Could you check a few things on this drawing? It's one solid part, dimensions in mm from its lowest x, y, z. Round coordinates to 2 decimals unless told otherwise and drop trailing zeros. Order: outer loops, then holes, each group sorted by start corner. A loop starts at its lowest first (then second) coordinate and runs counter-clockwise, first axis right, second up. Notation, with made-up numbers: M 30.25,76 L 60.25,76 A12 ccw 60.25,82 Z; hole C 0,-29 d10. An arc over 180 degrees is marked long. Answer as a JSON object with one key per item and string values. Group by question number.
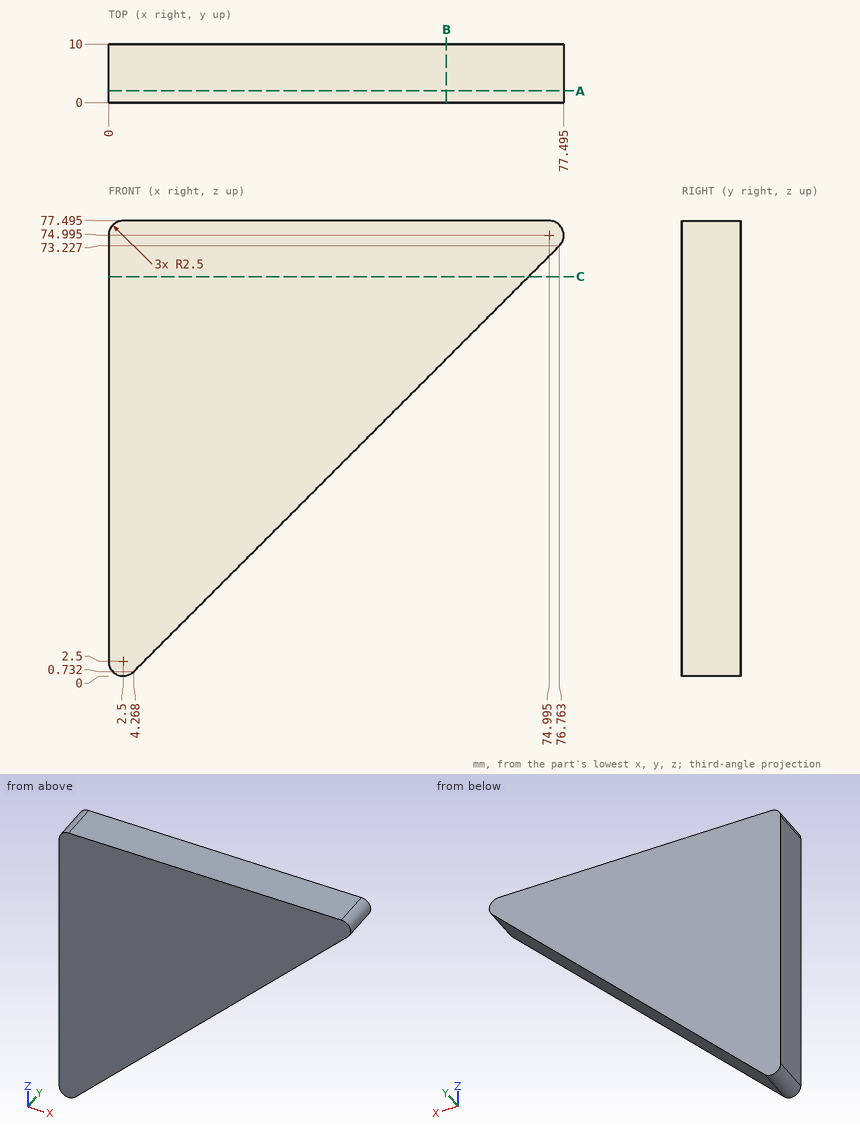
1) If we section it at C-C on z = 68: Write out the boundary of the cut face in (x, y) (1 decimal).
2) If we section it at B-B on x = 57.5: Write out the boundary of the cut face in (y, z) (1 decimal).
3) If we section it at A-A on y = 2: Write out the boundary of the cut face in (x, z) (1 decimal), plus the area to 3 significant figures.
4) I need wall thicknesses on line 1 along Z through (x, y) = (20.5, 6) (1 decimal); line 2 along Z through (x, y) = (27, 1) (1 decimal); line 3 along X through (y, z) = (4.25, 28.5) (1 decimal). Which ranges of each line are inside material? Lowest first, please.
5) For pin 1 (1 mm diameter, centred on y = 3, z = 8.5, fed in from +X) (1 decimal); pin 2 (1.5 mm diameter, centred on x = 49.5, y = 6.5, fed in from -Z) (1 decimal); pin 3 (2 mm diameter, centred on y = 3, z = 20.5, fed in from +X) (1 decimal), each with a flat end and sliding along its axis, tell me the tip position at first contact or that it passes through.
Findings:
{
 "1": {"outline": "M 0,0 L 71.5,0 L 71.5,10 L 0,10 Z"},
 "2": {"outline": "M 0,54 L 10,54 L 10,77.5 L 0,77.5 Z"},
 "3": {"outline": "M 0,2.5 A2.5 ccw 4.3,0.7 L 76.8,73.2 A2.5 ccw 75,77.5 L 2.5,77.5 A2.5 ccw 0,75 Z", "area": "3,270 mm^2"},
 "4": {"line 1": "z = 17 to 77.5", "line 2": "z = 23.5 to 77.5", "line 3": "x = 0 to 32"},
 "5": {"pin 1": "stops at x = 12.5", "pin 2": "stops at z = 45.2", "pin 3": "stops at x = 25"}
}
